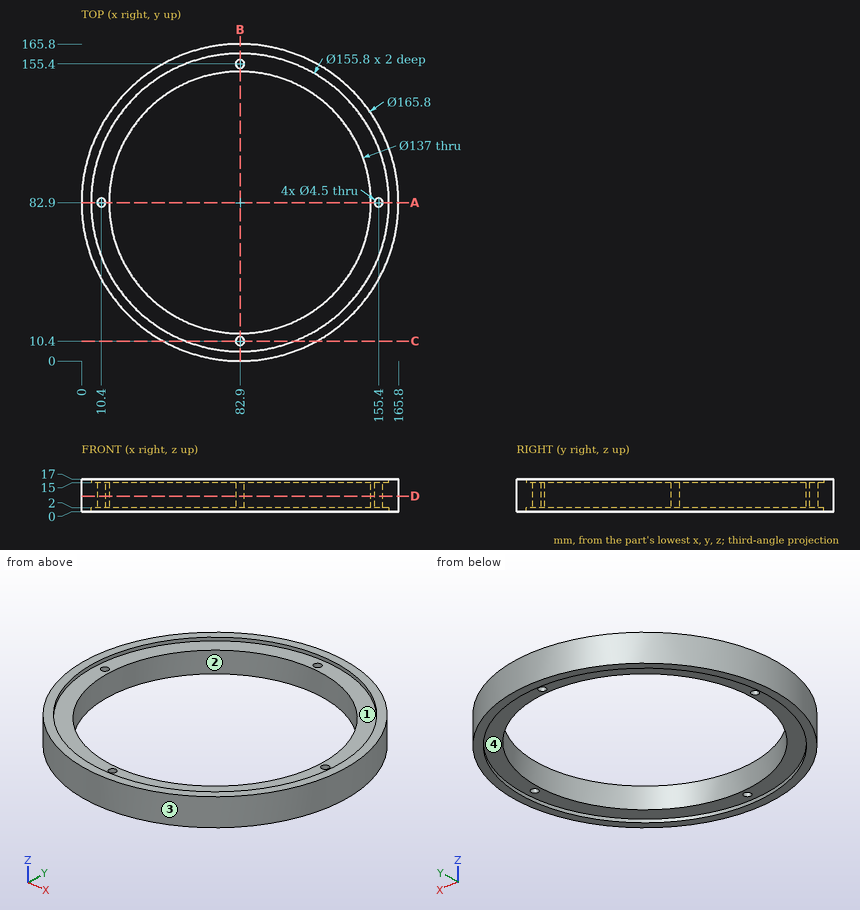
Study the drawing (mm; zero at the part's minimum x, y, z) and answer. A direction names the side the tool comes from. Give positions to 0.01 mm unless a question says otherwise; leave off trailing zeros. Write each loop counter-clockwise with the first axis right and the second up, starting at its lowest first coordinate (ties: lowest second). Pieces come first, ordered by that corner, then holes. Notation, with made-up numbers: (89.25, 77) - (100.25, 77) arc R3 ccw to (100.25, 81) - close; hole circle Ø1 at (-27, 23.5). An arc over 180 degrees is marked (long way). Write item = value, one per line. Start each with the question number.
Item 1: Each of these flat-tipped pins is pushed along its axis until it touches: P1, Ø2.5, axis at x = 155.4, y = 82.9, coming from the +Z side; P2, Ø5, axis at x = 82.9, y = 155.4, coming from the -Z side; P3, Ø6, axis at x = 87, z = 2.5, coming from the -Y side; P4, Ø3, axis at y = 76, z = 3.5, coming from the -X side. Where does it stop, or does it pass through?
Item 2: The mould has two halves that part along X. Classify the marked faces 3 and 4: +X half, -X half, draft (parallel to the pull), parting line (faces both ways), or undercut.
Item 3: Find the intervals of material crossed by probe 1 along Y at (x, z) = (82.9, 1.1); probe 2 along Y at (x, z) = (70, 8); probe 3 along X at (y, z) = (107.5, 11.25), in increasing order. Write a range as [from, to].
Item 4: Find section A-A (y = 82.9). Give the vertices of the cut face in (x, z).
Item 5: Find section D-D (z = 8). Give the vertices of the cut face in (x, y), then the cut area to 3 significant figures.
Item 6: A tool of negligible diameter and unlimited length cuts with its end or side. For the marked faces 1 and 2, from which of +Z, -Z, +X, -X, +Y, -Y can it reach the whole face along a straight path? Write none if from no direction.
Item 7: Find section C-C (y = 10.4). Give the vertices of the cut face in (x, z).
Response:
q1.P1 = through
q1.P2 = 2
q1.P3 = 0.01
q1.P4 = 0.18
q2.face_3 = parting line
q2.face_4 = undercut
q3.probe_1 = [0, 5], [160.8, 165.8]
q3.probe_2 = [1.01, 15.63], [150.17, 164.79]
q3.probe_3 = [3.73, 18.97], [146.83, 162.07]
q4.outline = (0, 0) - (5, 0) - (5, 2) - (8.15, 2) - (8.15, 15) - (5, 15) - (5, 17) - (0, 17) - close; (12.65, 2) - (14.4, 2) - (14.4, 15) - (12.65, 15) - close; (151.4, 2) - (153.15, 2) - (153.15, 15) - (151.4, 15) - close; (157.65, 2) - (160.8, 2) - (160.8, 0) - (165.8, 0) - (165.8, 17) - (160.8, 17) - (160.8, 15) - (157.65, 15) - close
q5.outline = circle Ø165.8 at (82.9, 82.9); hole circle Ø4.5 at (10.4, 82.9); hole circle Ø137 at (82.9, 82.9); hole circle Ø4.5 at (82.9, 10.4); hole circle Ø4.5 at (82.9, 155.4); hole circle Ø4.5 at (155.4, 82.9)
q5.area = 6,790 mm²
q6.face_1 = +Z
q6.face_2 = +Z, -Z
q7.outline = (42.7, 0) - (54.4, 0) - (54.4, 2) - (80.65, 2) - (80.65, 15) - (54.4, 15) - (54.4, 17) - (42.7, 17) - close; (85.15, 2) - (111.4, 2) - (111.4, 0) - (123.1, 0) - (123.1, 17) - (111.4, 17) - (111.4, 15) - (85.15, 15) - close
